from build123d import *

# Parameters (mm, degrees)
BOSS_EXTRUDE2_DEPTH = 12.7
SKETCH6_R           = 12.7
BOSS_EXTRUDE3_DEPTH = 57.15
SKETCH10_R          = 12.7
BOSS_EXTRUDE5_DEPTH = 6.35
CHAMFER2_SIZE       = 6.35


with BuildPart() as part:
    # Sketch5 → Boss-Extrude2 (new body)
    with BuildSketch(Plane(origin=(0, 0, 0), x_dir=(1, 0, 0), z_dir=(0, 1, 0))):
        Polygon((19.247414599, 0), (9.6237073, 16.66875), (-9.6237073, 16.66875), (-19.247414599, 0), (-9.6237073, -16.66875), (9.6237073, -16.66875), align=None)
    extrude(amount=BOSS_EXTRUDE2_DEPTH)

    # Sketch6 → Boss-Extrude3 (add)
    with BuildSketch(Plane.XZ):
        with Locations(Location((0, 0, 0), (0, 0, 270))):
            Circle(SKETCH6_R)
    extrude(amount=BOSS_EXTRUDE3_DEPTH)

    # Sketch10 → Boss-Extrude5 (add)
    with BuildSketch(Plane.XZ.offset(57.15)):
        with Locations(Location((0, 0, 0), (0, 0, 270))):
            Circle(SKETCH10_R)
    extrude(amount=BOSS_EXTRUDE5_DEPTH)

    # Chamfer2
    chamfer2_edges = [part.edges().sort_by_distance(p)[0] for p in [
        (0, -63.5, 12.7),
    ]]
    chamfer(chamfer2_edges, length=CHAMFER2_SIZE)


solid = part.part
Here's how the part is built. I have some questions about the finished solid (model axes, mm). A direction names the side the tool comes from. Round coordinates to 2 decimals unless told otherwise and drop trailing zeros. Order: outer loops, then holes, each group sorted by start corner. A loop starts at its lowest first (then second) coordinate and runs counter-clockwise, first axis right, second up. Notation, with made-up numbers: (64, -29) -> (101, -29) arc R16 cw to (101, -24) -> close; hole circle Ø11 at (70.5, -4). An arc over 180 degrees is marked (long way). Use CSV: the item, a comma, the result in double quotes.
1. I want a section at C-C on y = -59. List the corners of the cut face in (x, z) for me, and give its area (3 significant figures).
Recorded:
outline,"circle Ø21.7 at (0, 0)"
area,"370 mm2"
2. Which directions (+Z, -Z, +X, -X, +Y, -Y) give clear straight access to the entire face, cutting with the end or side of a thin tool? Please do faces 1 (the face through (-7.7, -28.2, 10.1)), 2 (the face through (0, 6, 16.669)).
Recorded:
face 1,"-Y"
face 2,"+Z, +X, -X, +Y, -Y"
3. I'm going to push flat-ended pins straight in: P1, Ø3, axis at x = 8, y = -35, coming from the +Z side; P2, Ø2, axis at x = 6.5, y = -18.5, coming from the +Z side; P3, Ø12, axis at x = -14, z = -6, coming from the -Y side. Where does each tip first touch, or does it pass through?
Recorded:
P1,"stops at z = 10.91"
P2,"stops at z = 11.45"
P3,"stops at y = -60.62"
4. I want a section at B-B on y = -23. List the corners of the cut face in (x, z) for me, and give its area (3 significant figures).
Recorded:
outline,"circle Ø25.4 at (0, 0)"
area,"507 mm2"
5. I want a section at A-A on x = 0. List the corners of the cut face in (y, z) for me.
Recorded:
outline,"(-63.5, -6.35) -> (-57.15, -12.7) -> (0, -12.7) -> (0, -16.67) -> (12.7, -16.67) -> (12.7, 16.67) -> (0, 16.67) -> (0, 12.7) -> (-57.15, 12.7) -> (-63.5, 6.35) -> close"
6. I need wall thicknesses on line 1 along X through (y, z) = (-8, -11); line 2 along Y through (x, z) = (10.5, -12.5); line 3 along X through (y, z) = (-51, -0.5). Which ranges of each line are inside material? Lowest first, please.
Recorded:
line 1,"x = -6.35 to 6.35"
line 2,"y = 0 to 12.7"
line 3,"x = -12.69 to 12.69"
